Can you work these out from the drawing? Everything is in mm from the part's minimum corner. Round coordinates to 2 decimals unless told otherwise and drop trailing zeros. Order: outer loops, then holes, each group sorted by start corner. A loop starts at its lowest first (then second) coordinate and runs counter-clockwise, first axis right, second up. Notation, with made-up numbers: (-14, -6) -> (45, -6) arc R20 cw to (45, 25) -> close; hole circle Ø10 at (-15.5, 1.5). An arc over 180 degrees is marked (long way). Use a Markdown table: item, result. Add a question column.
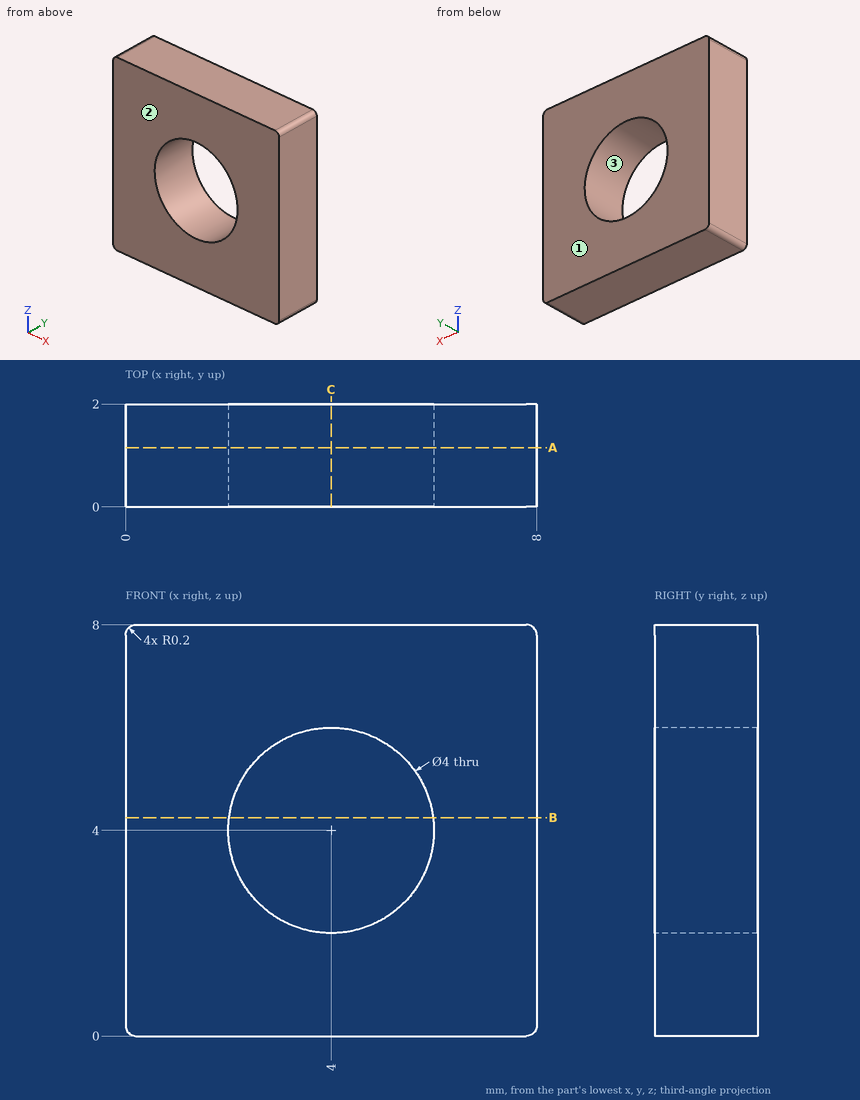
(1) If we mould it in two halves opening along Y, with no side actions, what happens to the marked faces 1, 2 and 3? For each: pulls with the +Y half, pulls with the -Y half, needs draft (parallel to the pull), parting line crosses it, or undercut.
(2) I want a section at A-A on y = 1.15. List the corners of the cut face in (x, z) for me.
(3) I want a section at B-B on z = 4.25. List the corners of the cut face in (x, y) for me.
(4) Please list where these lines run through material, in increasing order: probe 1 along X at (y, z) = (0.5, 4); probe 2 along Z at (x, y) = (3.25, 0.4); probe 3 along X at (y, z) = (0.6, 5.5). Write a range as from..to.
(5) I want a section at C-C on x = 4. List the corners of the cut face in (y, z) for me, and give its area (3 significant figures).
Output:
| question | item | result |
|---|---|---|
| 1 | face 1 | pulls with the +Y half |
| 1 | face 2 | pulls with the -Y half |
| 1 | face 3 | needs draft |
| 2 | outline | (0, 0.2) arc R0.2 ccw to (0.2, 0) -> (7.8, 0) arc R0.2 ccw to (8, 0.2) -> (8, 7.8) arc R0.2 ccw to (7.8, 8) -> (0.2, 8) arc R0.2 ccw to (0, 7.8) -> close; hole circle Ø4 at (4, 4) |
| 3 | outline | (0, 0) -> (2.02, 0) -> (2.02, 2) -> (0, 2) -> close; (5.98, 0) -> (8, 0) -> (8, 2) -> (5.98, 2) -> close |
| 4 | probe 1 | 0..2, 6..8 |
| 4 | probe 2 | 0..2.15, 5.85..8 |
| 4 | probe 3 | 0..2.68, 5.32..8 |
| 5 | outline | (0, 0) -> (2, 0) -> (2, 2) -> (0, 2) -> close; (0, 6) -> (2, 6) -> (2, 8) -> (0, 8) -> close |
| 5 | area | 8.00 mm² |
